Could you check a few things on this drawing? It's one solid part, dimensions in mm from its lowest x, y, z. Give positions to 0.01 mm unless a question says otherwise; leave off trailing zeros. Loops run counter-clockwise (first coordinate to the right, second up) from the corner with the lowest first, then second, coordinate; pieces in that order, holes last. Notation, with made-up numbers: (14.25, -1) - (32.25, -1) arc R7 ccw to (32.25, 3) - close; hole circle Ø9 at (43, 30.5). An arc over 180 degrees is marked (long way). Write item = value, one per line.
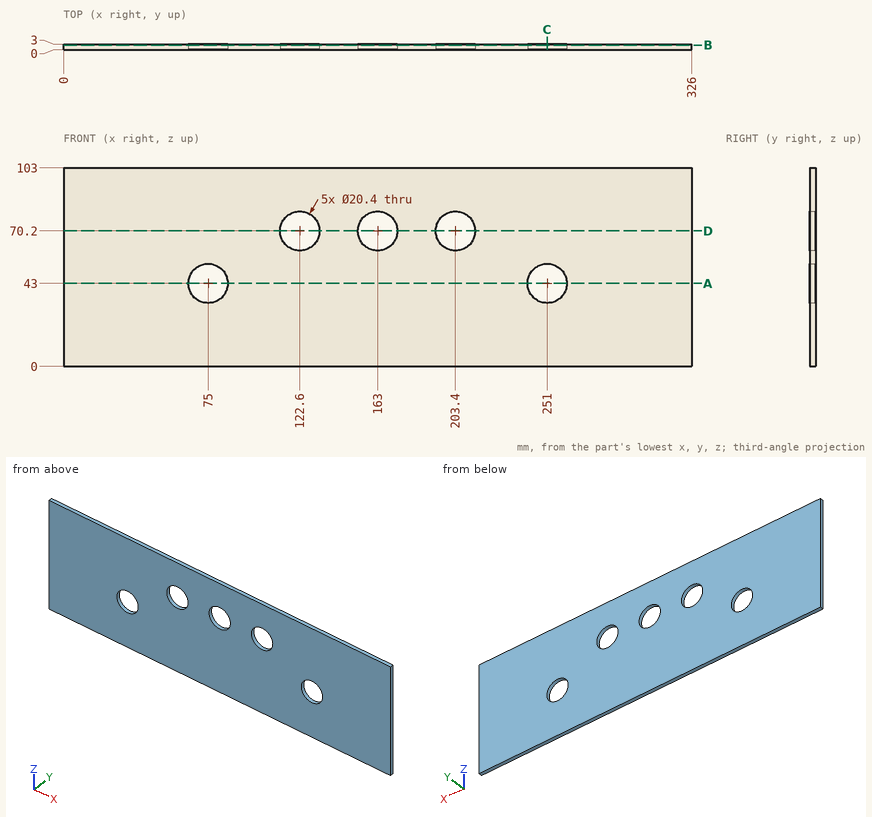
Q1. Imagine slicing it at B-B, the plane y = 2.4. Write out the boundary of the cut face in (x, z).
Output:
outline = (0, 0) - (326, 0) - (326, 103) - (0, 103) - close; hole circle Ø20.4 at (75, 43); hole circle Ø20.4 at (122.6, 70.2); hole circle Ø20.4 at (163, 70.2); hole circle Ø20.4 at (203.4, 70.2); hole circle Ø20.4 at (251, 43)
Q2. I need wall thicknesses on L1, parallel to X at y = 2.1, z = 70.2; L2, parallel to X at y = 1.65, z = 41; L3, parallel to X at y = 2.05, z = 64.5. Which ranges of each line are inside material? Lowest first, please.
Output:
L1 = 0 to 112.4, 132.8 to 152.8, 173.2 to 193.2, 213.6 to 326
L2 = 0 to 65, 85 to 241, 261 to 326
L3 = 0 to 114.14, 131.06 to 154.54, 171.46 to 194.94, 211.86 to 326
Q3. Imagine slicing it at C-C, the plane x = 251. Write out the boundary of the cut face in (y, z).
Output:
outline = (0, 0) - (3, 0) - (3, 32.8) - (0, 32.8) - close; (0, 53.2) - (3, 53.2) - (3, 103) - (0, 103) - close
Q4. Imagine slicing it at D-D, the plane z = 70.2. Write out the boundary of the cut face in (x, y), then the cut area to 3 significant figures.
Output:
outline = (0, 0) - (112.4, 0) - (112.4, 3) - (0, 3) - close; (132.8, 0) - (152.8, 0) - (152.8, 3) - (132.8, 3) - close; (173.2, 0) - (193.2, 0) - (193.2, 3) - (173.2, 3) - close; (213.6, 0) - (326, 0) - (326, 3) - (213.6, 3) - close
area = 794 mm2
Q5. Imagine slicing it at A-A, the plane z = 43. Write out the boundary of the cut face in (x, y), then the cut area to 3 significant figures.
Output:
outline = (0, 0) - (64.8, 0) - (64.8, 3) - (0, 3) - close; (85.2, 0) - (240.8, 0) - (240.8, 3) - (85.2, 3) - close; (261.2, 0) - (326, 0) - (326, 3) - (261.2, 3) - close
area = 856 mm2
Q6. For pin 1 (12 mm diameter, centred on x = 203.4, z = 70.2, fed in from -Y); pin 2 (23.5 mm diameter, centred on x = 251, z = 43, fed in from -Y), each with a flat end and sliding along its axis, tell me the tip position at first contact or that it passes through.
Output:
pin_1 = through
pin_2 = 0
